```python
from build123d import *

# Parameters (mm, degrees)
SKETCH1_R           = 2.5
BOSS_EXTRUDE1_DEPTH = 20
SKETCH2_R           = 2.5
CUT_EXTRUDE1_DEPTH  = 12.5
CUT_EXTRUDE2_DEPTH  = 5
FILLET5_R           = 10
FILLET6_R           = 10
FILLET7_R           = 10
FILLET8_R           = 10
FILLET9_R           = 5


with BuildPart() as part:
    # Sketch1 → Boss-Extrude1 (new body)
    with BuildSketch(Plane.XY):
        with BuildLine():
            ThreePointArc((26.829629131, 51.705904774), (18.464466094, 56.535533906), (23.294095226, 48.170370869))
            Line((23.294095226, 48.170370869), (52.0520382, 19.412427894))
            Line((52.0520382, 19.412427894), (52.0520382, -27.9479618))
            Line((52.0520382, -27.9479618), (25, -55))
            Line((25, -55), (0, -55))
            Line((0, -55), (0, -60))
            Line((0, -60), (27.071067812, -60))
            Line((27.071067812, -60), (57.0520382, -30.019029611))
            Line((57.0520382, -30.019029611), (57.0520382, 21.483495706))
            Line((57.0520382, 21.483495706), (26.829629131, 51.705904774))
        make_face()
        with Locations((22, 53)):
            Circle(SKETCH1_R, mode=Mode.SUBTRACT)
    boss_extrude1 = extrude(amount=BOSS_EXTRUDE1_DEPTH)

    # Sketch2 → Cut-Extrude1 (cut)
    with BuildSketch(Plane.XY.offset(20)):
        with BuildLine():
            ThreePointArc((23.294095226, 48.170370869), (25.535533906, 49.464466094), (26.829629131, 51.705904774))
            ThreePointArc((26.829629131, 51.705904774), (26.957224307, 52.347369039), (27, 53))
            ThreePointArc((27, 53), (18.033233299, 56.043807145), (23.294095226, 48.170370869))
        make_face()
        with Locations((22, 53)):
            Circle(SKETCH2_R, mode=Mode.SUBTRACT)
        with BuildLine():
            Line((41.940833666, 36.59470024), (26.829629131, 51.705904774))
            ThreePointArc((26.829629131, 51.705904774), (25.535533906, 49.464466094), (23.294095226, 48.170370869))
            Line((23.294095226, 48.170370869), (37.673066713, 33.791399381))
            Line((37.673066713, 33.791399381), (41.940833666, 36.59470024))
        make_face()
    cut_extrude1 = extrude(amount=-CUT_EXTRUDE1_DEPTH, mode=Mode.SUBTRACT)

    # Sketch3 → Cut-Extrude2 (cut)
    with BuildSketch(Plane(origin=(0, -55, 0), x_dir=(1, 0, 0), z_dir=(0, 1, 0))):
        Polygon((25, -20), (0, 0), (0, -20), align=None)
    cut_extrude2 = extrude(amount=-CUT_EXTRUDE2_DEPTH, mode=Mode.SUBTRACT)

    # Mirror2: Boss-Extrude1, Cut-Extrude1, Cut-Extrude2 across plane
    add(boss_extrude1.mirror(Plane.XY))
    add(cut_extrude1.mirror(Plane.XY), mode=Mode.SUBTRACT)
    add(cut_extrude2.mirror(Plane.XY), mode=Mode.SUBTRACT)

    # Fillet5
    fillet5_edges = [part.edges().sort_by_distance(p)[0] for p in [
        (39.806950189, 35.193049811, -20),
        (39.806950189, 35.193049811, 20),
    ]]
    fillet(fillet5_edges, radius=FILLET5_R)

    # Fillet6
    fillet6_edges = [part.edges().sort_by_distance(p)[0] for p in [
        (27.071067812, -60, 0),
        (57.0520382, -30.019029611, 0),
        (57.0520382, 21.483495706, 0),
    ]]
    fillet(fillet6_edges, radius=FILLET6_R)

    # Fillet7
    fillet7_edges = [part.edges().sort_by_distance(p)[0] for p in [
        (25, -55, 0),
        (52.0520382, -27.9479618, 0),
        (52.0520382, 19.412427894, 0),
    ]]
    fillet(fillet7_edges, radius=FILLET7_R)

    # Fillet8
    fillet8_edges = [part.edges().sort_by_distance(p)[0] for p in [
        (25, -56.942490323, -20),
        (25, -56.942490323, 20),
    ]]
    fillet(fillet8_edges, radius=FILLET8_R)

    # Fillet9
    fillet9_edges = [part.edges().sort_by_distance(p)[0] for p in [
        (0, -57.5, 0),
    ]]
    fillet(fillet9_edges, radius=FILLET9_R)


solid = part.part
```
Geometry: final body of the model. Coordinates: model frame, mm. A direction names the side the tool comes from. Coordinates: 2 decimals unless noted, no trailing zeros. Order: outer loops, then holes, each group sorted by start corner. A loop starts at its lowest first (then second) coordinate and runs counter-clockwise, first axis right, second up. Notation, with made-up numbers: (8.5, 46) - (30.5, 46) arc R24 cw to (30.5, 71) - close; hole circle Ø3 at (21, 50). An arc over 180 degrees is marked (long way). Write each question's results on one line, items separated by ' | '.
1) Section B-B, the plane z = 2. Return loops of the section in (x, y).
Results list:
outline: (3.42, -60) - (22.93, -60) arc R10 ccw to (30, -57.07) - (54.12, -32.95) arc R10 ccw to (57.05, -25.88) - (57.05, 17.34) arc R10 ccw to (54.12, 24.41) - (26.83, 51.71) arc R5 ccw (long way) to (23.29, 48.17) - (49.12, 22.34) arc R10 cw to (52.05, 15.27) - (52.05, -23.81) arc R10 cw to (49.12, -30.88) - (27.93, -52.07) arc R10 cw to (20.86, -55) - (3.42, -55) - close; hole circle Ø5 at (22, 53)
2) Set-up query: faces 1 (the flat face through (52.23, -14.26, -20)), 2 (the cylindrical face through (51.312, -27.582, 0.28)). Return all of +Z, -Z, +X, -X, +Y, -Y with unobstructed straight access to the full face (end or side cutting, diameter ignored); none if empty.
Results list:
face 1: -Z, +X, -X, +Y, -Y | face 2: +Z, -Z, -X
3) Section C-C, the plane x = 10. Return loops of the section in (y, z), plus the area to 3 significant figures.
Results list:
outline: (-60, -8) - (-55, -8) - (-55, 8) - (-60, 8) - close | area: 80.0 mm^2
4) Line query: line 1 (Y direction, x = 22, z = 1.5); line 2 (Y direction, x = 21, z = -6.5); line 3 (X direction, y = 51.5, z = 3). Output: solid intervals per line, ascending. Write a range as from..to.
Results list:
line 1: -60..-54.93, 48..50.5, 55.5..58 | line 2: -60..-55, 48.1..50.71, 55.29..57.9 | line 3: 17.23..20, 24..27.04
5) Pull-direction query (Y, two-part tool) for faces 3 (the cylindrical face through (42.28, 33.41, -16.99)), 4 (the flat face through (39, -41, 0)), 5 (the cylindrical face through (3.004, -57.535, 0.063)); classes: pulls with the +Y half, pulls with the -Y half, needs draft (parallel to the pull), parting line crosses it, or undercut.
Results list:
face 3: pulls with the +Y half | face 4: undercut | face 5: needs draft
6) Section A-A, the plane y = 53. Return loops of the section in (x, z).
Results list:
outline: (17, -7.5) - (19.5, -7.5) - (19.5, 7.5) - (17, 7.5) - close; (24.5, -7.5) - (27, -7.5) - (27, 7.5) - (24.5, 7.5) - close
7) Section D-D, the plane z = -12.5. Return loops of the section in (x, y) (3 decimals).
Results list:
outline: (15.625, -60) - (22.929, -60) arc R10 ccw to (30, -57.071) - (54.123, -32.948) arc R10 ccw to (57.052, -25.877) - (57.052, 17.341) arc R10 ccw to (54.123, 24.412) - (42.17, 36.365) - (37.902, 33.562) - (49.123, 22.341) arc R10 cw to (52.052, 15.27) - (52.052, -23.806) arc R10 cw to (49.123, -30.877) - (27.929, -52.071) arc R10 cw to (20.858, -55) - (15.625, -55) - close
8) Pin query (flat end, axial travel): pin 1 (8 mm diameter, centred on x = 9, z = 1, fed in from +Y); pin 2 (1 mm diameter, centred on x = 35, z = -7, fed in from +Y); pin 3 (1.5 mm diameter, centred on x = 28, z = 1, fed in from -Y). Return the tip coordinate at first contact, or that it passes through.
Results list:
pin 1: y = -55 | pin 2: y = 44.04 | pin 3: y = -59.02
